```python
from build123d import *

# Parameters (mm, degrees)
SKETCH1_W           = 53.975
SKETCH1_H           = 88.9
SKETCH1_R           = 7.9375
SKETCH1_R_2         = 17.4625
BOSS_EXTRUDE1_DEPTH = 50.8
SKETCH5_R           = 2.09
CUT_EXTRUDE1_DEPTH  = 116.746060948
SKETCH5_3_R         = 3.6
CUT_EXTRUDE2_DEPTH  = 4.064
CUT_EXTRUDE3_DEPTH  = 2.54
FILLET1_R           = 1.27


with BuildPart() as part:
    # Sketch1 → Boss-Extrude1 (new body)
    with BuildSketch(Plane(origin=(0, 0, 0), x_dir=(0, 0, -1), z_dir=(1, 0, 0))):
        with Locations((26.9875, 44.45)):
            Rectangle(SKETCH1_W, SKETCH1_H)
        with Locations(Location((26.9875, 19.685, 0), (0, 0, 180))):
            Circle(SKETCH1_R, mode=Mode.SUBTRACT)
        with Locations(Location((26.9875, 60.325, 0), (0, 0, 180))):
            Circle(SKETCH1_R_2, mode=Mode.SUBTRACT)
    extrude(amount=BOSS_EXTRUDE1_DEPTH)

    # Sketch5 → Cut-Extrude1 (cut, through all)
    with BuildSketch(Plane.XY):
        with Locations((12.7, 83.34375)):
            Circle(SKETCH5_R)
        with Locations((12.7, 35.2425)):
            Circle(SKETCH5_R)
        with Locations((38.1, 83.34375)):
            Circle(SKETCH5_R)
        with Locations((38.1, 35.2425)):
            Circle(SKETCH5_R)
        with Locations((12.7, 5.87375)):
            Circle(SKETCH5_R)
        with Locations((38.1, 5.87375)):
            Circle(SKETCH5_R)
    extrude(amount=-CUT_EXTRUDE1_DEPTH, mode=Mode.SUBTRACT)

    # Sketch5<3> → Cut-Extrude2 (cut)
    with BuildSketch(Plane.XY):
        with Locations((38.1, 35.2425)):
            Circle(SKETCH5_3_R)
        with Locations((12.7, 83.34375)):
            Circle(SKETCH5_3_R)
        with Locations((38.1, 83.34375)):
            Circle(SKETCH5_3_R)
        with Locations((12.7, 35.2425)):
            Circle(SKETCH5_3_R)
        with Locations((38.1, 5.87375)):
            Circle(SKETCH5_3_R)
        with Locations((12.7, 5.87375)):
            Circle(SKETCH5_3_R)
    extrude(amount=-CUT_EXTRUDE2_DEPTH, mode=Mode.SUBTRACT)

    # Sketch6 → Cut-Extrude3 (cut)
    with BuildSketch(Plane(origin=(0, 0, -53.975), x_dir=(-1, 0, 0), z_dir=(0, 0, -1))):
        Polygon((-34.02855, 83.34375), (-36.064275, 86.86972913), (-40.135725, 86.86972913), (-42.17145, 83.34375), (-40.135725, 79.81777087), (-36.064275, 79.81777087), align=None)
        Polygon((-8.62855, 83.34375), (-10.664275, 86.86972913), (-14.735725, 86.86972913), (-16.77145, 83.34375), (-14.735725, 79.81777087), (-10.664275, 79.81777087), align=None)
        Polygon((-8.62855, 35.2425), (-10.664275, 38.76847913), (-14.735725, 38.76847913), (-16.77145, 35.2425), (-14.735725, 31.71652087), (-10.664275, 31.71652087), align=None)
        Polygon((-34.02855, 35.2425), (-36.064275, 38.76847913), (-40.135725, 38.76847913), (-42.17145, 35.2425), (-40.135725, 31.71652087), (-36.064275, 31.71652087), align=None)
        Polygon((-34.02855, 5.87375), (-36.064275, 9.39972913), (-40.135725, 9.39972913), (-42.17145, 5.87375), (-40.135725, 2.34777087), (-36.064275, 2.34777087), align=None)
        Polygon((-8.62855, 5.87375), (-10.664275, 9.39972913), (-14.735725, 9.39972913), (-16.77145, 5.87375), (-14.735725, 2.34777087), (-10.664275, 2.34777087), align=None)
    extrude(amount=-CUT_EXTRUDE3_DEPTH, mode=Mode.SUBTRACT)

    # Fillet1
    fillet1_edges = [part.edges().sort_by_distance(p)[0] for p in [
        (0, 60.325, -44.45),
        (50.8, 60.325, -44.45),
        (50.8, 88.9, -26.9875),
        (0, 19.685, -34.925),
        (50.8, 19.685, -34.925),
        (50.8, 44.45, 0),
        (50.8, 0, -26.9875),
        (0, 44.45, 0),
        (0, 88.9, -26.9875),
        (0, 44.45, -53.975),
        (0, 0, -26.9875),
        (25.4, 0, 0),
        (25.4, 88.9, 0),
        (25.4, 88.9, -53.975),
        (25.4, 0, -53.975),
        (50.8, 44.45, -53.975),
    ]]
    fillet(fillet1_edges, radius=FILLET1_R)

    # SurfaceCut1
    split(bisect_by=Plane.XY.offset(-26.9875), keep=Keep.TOP)


solid = part.part
```
For this review, take the finished solid that the model builds, in its own axes (mm). A direction names the side the tool comes from. Round coordinates to 2 decimals unless told otherwise and drop trailing zeros. Write each loop counter-clockwise with the first axis right and the second up, starting at its lowest first coordinate (ties: lowest second). Pieces come first, ordered by that corner, then holes. Notation, with made-up numbers: (-23, 0) - (35, 0) arc R24 ccw to (35, 38) - close; hole circle Ø1 at (-1, 5.5). An arc over 180 degrees is marked (long way). Answer as a JSON object with one key per item and string values.
1. Tool access review of faces 5 (the face through (25, 0, -14)), 6 (the face through (37.32, 2.36, -2)): name each direction out of +Z, -Z, +X, -X, +Y, -Y from which nothing blocks a thin tool from reaching the whole face with its end or side.
Response values:
{"face 5": "+Z, -Z, +X, -X, -Y", "face 6": "+Z"}
2. We need section A-A on x = 38.1. Count the separate pieces of the cut face and the enclosed holes in it, then the cut area to 3 significant figures.
Response values:
{"separate pieces": "4", "enclosed holes": "0", "area": "1,450 mm2"}
3. To check wall thickness, follow line 1 along Y through (x, z) = (12.7, -1.1); line 2 along X through (y, z) = (84, -15.25); line 3 along Y through (x, z) = (48.5, -20.5). State the ranges of each line that lie inside material, in increasing order.
Response values:
{"line 1": "y = 0.01 to 2.27, 9.47 to 31.64, 38.84 to 79.74, 86.94 to 88.89", "line 2": "x = 0 to 10.72, 14.68 to 36.12, 40.08 to 50.8", "line 3": "y = 0 to 15.11, 24.26 to 44.11, 76.54 to 88.9"}
4. We need section B-B on z = -6.5. Give the boundary of the cut face in (x, y).
Response values:
{"outline": "(0, 1.27) arc R1.27 ccw to (1.27, 0) - (49.53, 0) arc R1.27 ccw to (50.8, 1.27) - (50.8, 87.63) arc R1.27 ccw to (49.53, 88.9) - (1.27, 88.9) arc R1.27 ccw to (0, 87.63) - close; hole circle Ø4.18 at (12.7, 5.87); hole circle Ø4.18 at (12.7, 35.24); hole circle Ø4.18 at (12.7, 83.34); hole circle Ø4.18 at (38.1, 5.87); hole circle Ø4.18 at (38.1, 35.24); hole circle Ø4.18 at (38.1, 83.34)"}
5. Draft analysis for pull direction X (two halves, no side actions). For faces 1 (the face through (14.63, 82.54, -15.37)), 2 (the face through (40, 4, -4.064)), 3 (the face through (50.8, 45, -11)), 4 (the face through (25, 88.9, -14)), state which applies: +X half, -X half, draft (parallel to the pull), parting line (faces both ways), or undercut.
Response values:
{"face 1": "undercut", "face 2": "undercut", "face 3": "+X half", "face 4": "draft"}
6. For pin 1 Ø12 at (x, y) = (22, 59) entering from -Z; pin 2 Ø6 at (x, y) = (38.1, 35.24) entering from +Z, all flat-tipped, find the tip position at first contact; note any pin that passes through.
Response values:
{"pin 1": "stops at z = -11.14", "pin 2": "stops at z = -4.06"}
